from build123d import *

# Parameters (mm, degrees)
SKETCH1_W           = 40
SKETCH1_H           = 100
BOSS_EXTRUDE1_DEPTH = 3.18
SKETCH2_W           = 12.5
SKETCH2_H           = 3.18
CUT_EXTRUDE1_DEPTH  = 4.18
SKETCH3_R           = 1.4
CUT_EXTRUDE2_DEPTH  = 4.18


with BuildPart() as part:
    # Sketch1 → Boss-Extrude1 (new body)
    with BuildSketch(Plane(origin=(0, 0, 0), x_dir=(1, 0, 0), z_dir=(0, 1, 0))):
        Rectangle(SKETCH1_W, SKETCH1_H)
    extrude(amount=BOSS_EXTRUDE1_DEPTH)

    # Sketch2 → Cut-Extrude1 (cut, through all)
    with BuildSketch(Plane(origin=(0, 3.18, 0), x_dir=(1, 0, 0), z_dir=(0, 1, 0))):
        with Locations((13.75, 48.41)):
            Rectangle(SKETCH2_W, SKETCH2_H)
        with Locations((-13.75, 48.41)):
            Rectangle(SKETCH2_W, SKETCH2_H)
    cut_extrude1 = extrude(amount=-CUT_EXTRUDE1_DEPTH, mode=Mode.SUBTRACT)

    # Mirror1: Cut-Extrude1 across plane
    add(cut_extrude1.mirror(Plane.XY), mode=Mode.SUBTRACT)

    # Sketch3 → Cut-Extrude2 (cut, through all)
    with BuildSketch(Plane(origin=(0, 3.18, 0), x_dir=(1, 0, 0), z_dir=(0, 1, 0))):
        with Locations((-11.309610499, -12.180202037)):
            Circle(SKETCH3_R)
        with Locations((10.190389501, 1.569797963)):
            Circle(SKETCH3_R)
        with Locations((-11.309610499, 15.319797963)):
            Circle(SKETCH3_R)
    extrude(amount=-CUT_EXTRUDE2_DEPTH, mode=Mode.SUBTRACT)


solid = part.part
For this review, take the finished solid that the model builds, in its own axes (mm). A direction names the side the tool comes from. Coordinates: 2 decimals unless noted, no trailing zeros. Order: outer loops, then holes, each group sorted by start corner. A loop starts at its lowest first (then second) coordinate and runs counter-clockwise, first axis right, second up. Notation, with made-up numbers: (1, 10.5) - (40, 10.5) arc R12 cw to (40, 31.5) - close; hole circle Ø11 at (45, 16). An arc over 180 degrees is marked (long way). Use one line per item in the form item = value.
Q1. Consider section A-A (y = 1.9). Give the boundary of the cut face in (x, z).
Checked values:
outline = (-20, -46.82) - (-7.5, -46.82) - (-7.5, -50) - (7.5, -50) - (7.5, -46.82) - (20, -46.82) - (20, 46.82) - (7.5, 46.82) - (7.5, 50) - (-7.5, 50) - (-7.5, 46.82) - (-20, 46.82) - close; hole circle Ø2.8 at (-11.31, -15.32); hole circle Ø2.8 at (-11.31, 12.18); hole circle Ø2.8 at (10.19, -1.57)
Q2. For P1, Ø1.7, axis at x = -11.31, z = 12.18, coming from the -Y side; P2, Ø1, axis at y = 1, z = 48.5, coming from the -X side; P3, Ø1.5, axis at x = -8.5, y = 2, coming from the -Z side; P4, Ø1.5, axis at x = -13, y = 3, coming from the +Z side, all flat-tipped, find the tip position at first contact; note any pin that passes through.
Checked values:
P1 = through
P2 = -7.5
P3 = -46.82
P4 = 46.82
Q3. For faces 1 (the flat face through (-7.5, 2, 48)), 2 (the flat face through (0, 0, -1)), 3 (the flat face through (14, 2, 46.82)), 4 (the flat face through (-7.5, 2, -48)), 5 (the flat face through (14, 2, -46.82)), list the 3-axis set-ups (+Z, -Z, +X, -X, +Y, -Y) from which the entire face can be reached by the end or side of a thin tool; tool diameter is ignored.
Checked values:
face_1 = +Z, -X, +Y, -Y
face_2 = +Z, -Z, +X, -X, -Y
face_3 = +Z, +X, +Y, -Y
face_4 = -Z, -X, +Y, -Y
face_5 = -Z, +X, +Y, -Y
Q4. Draft analysis for pull direction Z (two halves, no side actions). For faces 6 (the cylindrical face through (9.9, 1.6, -0.2)), 7 (the flat face through (-14, 2, 46.82)), 8 (the flat face through (7.5, 2, 48)), state which applies: +Z half, -Z half, draft (parallel to the pull), parting line (faces both ways), or undercut.
Checked values:
face_6 = undercut
face_7 = +Z half
face_8 = draft
Q5. For probe 1 along Z at (x, y) = (-11, 1.15); probe 2 along Z at (x, y) = (-15, 2.15); probe 3 along Z at (x, y) = (-10.5, 0.2), list the stretches that pass through material, from the lowest coordinate up. Write a range as from..to.
Checked values:
probe_1 = -46.82..-16.69, -13.95..10.81, 13.55..46.82
probe_2 = -46.82..46.82
probe_3 = -46.82..-16.46, -14.18..11.04, 13.32..46.82
Q6. Consider section B-B (x = -14.5). Give the boundary of the cut face in (y, z), then the cut area to 3 significant figures.
Checked values:
outline = (0, -46.82) - (3.18, -46.82) - (3.18, 46.82) - (0, 46.82) - close
area = 298 mm2
